from build123d import *

# Parameters (mm, degrees)
F0_W        = 25.5065411329
F0_H        = 9.1286599636
F0_W_2      = 9.6656344831
F0_W_3      = 7.5177252293
F0_H_2      = 15.3039256111
F0_H_3      = 17.4518460408
F1_DEPTH    = 5.08
F2_R        = 2.54
F3_R        = 2.54
F4_W        = 86.313597858
F4_H        = 12.2866295278
F5_DEPTH    = 25.4
F6_T1_DEPTH = 77.6565983155


# Not quite as in the source:
# - a fillet or chamfer that OpenCascade refuses, or shapes differently, is made with other operations: its cross-section is extruded or revolved along the edge and cut away or added


with BuildPart() as f1:
    # F0 (on Front) → F1 (new body, symmetric)
    with BuildSketch(Plane.XZ):
        with Locations((-64.7060722113, 33.9639782906)):
            Rectangle(F0_W, F0_H)
        with Locations((-89.8098852485, 33.9639782906)):
            Rectangle(F0_W_2, F0_H)
        with Locations((-81.2182053924, 46.1802710779)):
            Rectangle(F0_W_3, F0_H_2)
        with Locations((-81.2182053924, 33.9639782906)):
            Rectangle(F0_W_3, F0_H)
        with Locations((-81.2182053924, 20.6737252884)):
            Rectangle(F0_W_3, F0_H_3)
    extrude(amount=F1_DEPTH, both=True)

    # F2
    f2_edges = [f1.edges().sort_by_distance(p)[0] for p in [
        (-64.706072, -5.08, 38.528308),
        (-89.809885, -5.08, 38.528308),
    ]]
    fillet(f2_edges, radius=F2_R)

    # F3
    f3_edges = [f1.edges().sort_by_distance(p)[0] for p in [
        (-64.706072, -5.08, 29.399648),
        (-89.809885, -5.08, 29.399648),
        (-89.809885, 5.08, 29.399648),
        (-64.706072, 5.08, 29.399648),
        (-64.706072, 5.08, 38.528308),
        (-89.809885, 5.08, 38.528308),
    ]]
    fillet(f3_edges, radius=F3_R)

    # F4 (on Front) → F5 (join)
    with BuildSketch(Plane.XZ):
        with Locations((-33.4874503314, 34.556152299)):
            Rectangle(F4_W, F4_H)
    extrude(amount=F5_DEPTH)

    # F6: chamfer of 10.16 on 2 edges, made by hand

    # F6_s2 → F6_t1 (cut)
    with BuildSketch(Plane.XZ.offset(-26.1282991577)):
        Polygon((-0.4906514025, 40.699467063), (9.6693485975, 30.539467063), (9.6693485975, 40.699467063), align=None)
        Polygon((9.6693485975, 38.5728375351), (-0.4906514025, 28.4128375351), (9.6693485975, 28.4128375351), align=None)
    extrude(amount=F6_T1_DEPTH, mode=Mode.SUBTRACT)


solid = f1.part
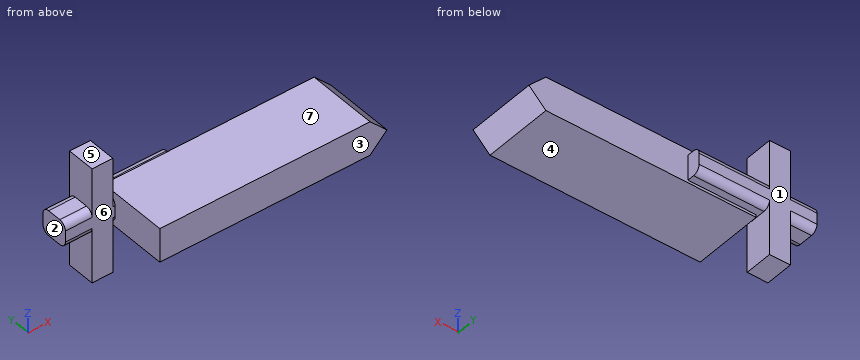
Could you check a few things on this model? Use its own coordinates, in mm. Face numbers are marked on the shaded views. A direction names the side the tool comes from. Give positions to 0.01 mm unless a question says otherwise; leave off trailing zeros. Loops run counter-clockwise (first coordinate to the right, second up) from the corner with the lowest first, then second, coordinate; pieces in that order, holes last. Notation, with made-up numbers: (70.5, -4) -> (112.5, -4) arc R12 ccw to (112.5, 0) -> close; hole circle Ø11 at (1.25, 3.5). An arc over 180 degrees is marked (long way). Return JSON: item names as keys, results as strings.
Item 1: We'd pull the mould along Y, two halves only. Please class the marked faces 1, 2 and 3: +Y half, -Y half, draft (parallel to the pull), parting line (faces both ways), or undercut.
Geometry results:
{"face 1": "+Y half", "face 2": "draft", "face 3": "-Y half"}
Item 2: I'm going to push flat-ended pins straight in: pin 1 (11 mm diameter, centred on y = -0.5, z = 47, fed in from -X); pin 2 (14.5 mm diameter, centred on x = -87, z = 30.5, fed in from -Y); pin 3 (6 mm diameter, centred on x = -55.5, y = -4, fed in from +Z). Where does each tip first touch, or does it pass through?
Geometry results:
{"pin 1": "stops at x = -84.98", "pin 2": "stops at y = -5.08", "pin 3": "stops at z = 40.7"}
Item 3: If we section it at D-D on y = -1: List the corners of the cut face in (x, z) for me, plus the area to 3 significant figures.
Geometry results:
{"outline": "(-94.64, 29.4) -> (-84.98, 29.4) -> (-84.98, 11.95) -> (-77.46, 11.95) -> (-77.46, 29.4) -> (-76.64, 29.4) -> (-76.64, 28.41) -> (-0.49, 28.41) -> (5.65, 34.56) -> (-0.49, 40.7) -> (-76.64, 40.7) -> (-76.64, 38.53) -> (-77.46, 38.53) -> (-77.46, 53.83) -> (-84.98, 53.83) -> (-84.98, 38.53) -> (-94.64, 38.53) -> close", "area": "1,380 mm²"}
Item 4: I need wall thicknesses on L1, parallel to Z at x = -74, y = -17.5; L2, parallel to Y at x = -4.5, z = 30; L3, parallel to X at y = 0.5, z = 25. Which ranges of each line are inside material? Lowest first, please. Write a range as from..to.
Geometry results:
{"L1": "z = 28.41..40.7", "L2": "y = -25.4..0", "L3": "x = -84.98..-77.46"}
Item 5: If we section it at A-A on y = -12.5: List the corners of the cut face in (x, z) for me.
Geometry results:
{"outline": "(-76.64, 28.41) -> (-0.49, 28.41) -> (5.65, 34.56) -> (-0.49, 40.7) -> (-76.64, 40.7) -> close"}
Item 6: Which directions (+Z, -Z, +X, -X, +Y, -Y) give clear straight access to the entire face, cutting with the end or side of a thin tool? Please do the marked faces 4, 5, 6 and 7.
Geometry results:
{"face 4": "-Z, +X, +Y, -Y", "face 5": "+Z, +X, -X, +Y, -Y", "face 6": "+Z, -Z, -X, -Y", "face 7": "+Z, +X, +Y, -Y"}
Item 7: If we section it at B-B on x = -53.5: List the corners of the cut face in (y, z) for me.
Geometry results:
{"outline": "(-25.4, 28.41) -> (0, 28.41) -> (0, 29.4) -> (2.54, 29.4) arc R2.54 ccw to (5.08, 31.94) -> (5.08, 35.99) arc R2.54 ccw to (2.54, 38.53) -> (0, 38.53) -> (0, 40.7) -> (-25.4, 40.7) -> close"}
Item 8: If we section it at C-C on z = 49.5: List the corners of the cut face in (x, y) for me.
Geometry results:
{"outline": "(-84.98, -5.08) -> (-77.46, -5.08) -> (-77.46, 5.08) -> (-84.98, 5.08) -> close"}
